Source: CAD feature listing. Evaluate the final solid. Frame: model axes, mm. Round coordinates to 2 decimals unless told otherwise and drop trailing zeros. Loops run counter-clockwise (first coordinate to the right, second up) from the corner with the lowest first, then second, coordinate; pieces in that order, holes last. Notation, with made-up numbers: (-15, 65.25) -> (-5, 65.25) arc R10 cw to (-5, 80.25) -> close; hole circle Ø2 at (48, -38). An arc over 180 degrees is marked (long way). Write item = value, one per line.
from build123d import *

# Parameters (mm, degrees)
F1_W     = 25.4
F1_H     = 25.4
F2_DEPTH = 25.4
F5_DEPTH = 25.4
F6_DEPTH = 25.4


with BuildPart() as f2:
    # F1 (on Top) → F2 (new body)
    with BuildSketch(Plane.XY):
        Rectangle(F1_W, F1_H)
    extrude(amount=F2_DEPTH)

    # F3 (on face) → F5 (cut)
    with BuildSketch(Plane.XZ.offset(12.7)):
        Polygon((-12.7, 25.4), (-12.7, 0), (0, 25.4), align=None)
        Polygon((12.7, 25.4), (0, 25.4), (12.7, 0), align=None)
    extrude(amount=-F5_DEPTH, mode=Mode.SUBTRACT)

    # F4 (on face) → F6 (cut)
    with BuildSketch(Plane.YZ.offset(12.7)):
        Polygon((-12.7, 25.4), (-12.7, 0), (0, 25.4), align=None)
        Polygon((12.7, 25.4), (0, 25.4), (12.7, 0), align=None)
    extrude(amount=-F6_DEPTH, mode=Mode.SUBTRACT)


solid = f2.part
1. Section query B-B (z = 12). Return the cut outline in (x, y), then the cut area to 3 significant figures.
Evaluation:
outline = (-6.7, -6.7) -> (6.7, -6.7) -> (6.7, 6.7) -> (-6.7, 6.7) -> close
area = 180 mm²
2. Line query: probe 1 along X at (y, z) = (9.25, 5); probe 2 along Z at (x, y) = (-10.5, 6); probe 3 along Z at (x, y) = (-6.25, -9.75). Output: solid intervals per line, ascending. Write a range as from..to.
Evaluation:
probe_1 = -10.2..10.2
probe_2 = 0..4.4
probe_3 = 0..5.9
3. Section query A-A (x = 11). Return the cut outline in (y, z).
Evaluation:
outline = (-12.7, 0) -> (12.7, 0) -> (11, 3.4) -> (-11, 3.4) -> close
4. Contact query for flat-ended pins moving along their axis: pin 1 Ø3 at (x, z) = (0, 22) entering from +Y; pin 2 Ø6 at (y, z) = (-10, 18) entering from +X; pin 3 Ø6 at (y, z) = (-7.5, 9.5) entering from +X; pin 4 Ø5 at (y, z) = (-10, 9) entering from -X. Output: stop coordinate, or through.
Evaluation:
pin_1 = 2.45
pin_2 = through
pin_3 = 9.45
pin_4 = -9.42
